The listing builds one solid part. Answer for the finished solid, in the listing's coordinates (mm). Face numbers are marked on the shaded views. A direction names the side the tool comes from. Coordinates: 2 decimals unless noted, no trailing zeros. Order: outer loops, then holes, each group sorted by start corner. A loop starts at its lowest first (then second) coordinate and runs counter-clockwise, first axis right, second up.
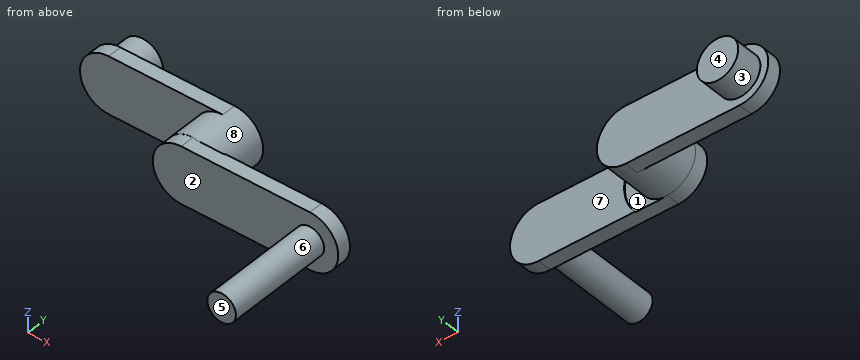
from build123d import *

# Parameters (mm, degrees)
SKETCH1_R           = 30
BOSS_EXTRUDE1_DEPTH = 25.4
BOSS_EXTRUDE2_DEPTH = 10
SKETCH3_R           = 14.5
BOSS_EXTRUDE3_DEPTH = 18.864779219
BOSS_EXTRUDE4_DEPTH = 10
SKETCH5_R           = 10
BOSS_EXTRUDE5_DEPTH = 75
CUT_EXTRUDE1_START  = -26
SKETCH7_R           = 30
SKETCH7_R_2         = 20
CUT_EXTRUDE1_DEPTH  = 26


with BuildPart() as part:
    # Sketch1 → Boss-Extrude1 (new body)
    with BuildSketch(Plane(origin=(0, 0, 0), x_dir=(1, 0, 0), z_dir=(0, 1, 0))):
        with Locations(Location((0, 0, 0), (0, 0, 270))):
            Circle(SKETCH1_R)
    extrude(amount=BOSS_EXTRUDE1_DEPTH)

    # Sketch2 → Boss-Extrude2 (add)
    with BuildSketch(Plane(origin=(0, 25.4, 0), x_dir=(1, 0, 0), z_dir=(0, 1, 0))):
        with BuildLine():
            Line((0, -20), (-80, -20))
            ThreePointArc((-80, -20), (-100, 0), (-80, 20))
            Line((-80, 20), (0, 20))
            ThreePointArc((0, 20), (20, 0), (0, -20))
        make_face()
    extrude(amount=BOSS_EXTRUDE2_DEPTH)

    # Sketch3 → Boss-Extrude3 (add)
    with BuildSketch(Plane(origin=(0, 35.4, 0), x_dir=(1, 0, 0), z_dir=(0, 1, 0))):
        with Locations(Location((-80, 0, 0), (0, 0, 270))):
            Circle(SKETCH3_R)
    extrude(amount=BOSS_EXTRUDE3_DEPTH)

    # Sketch4 → Boss-Extrude4 (add)
    with BuildSketch(Plane.XZ):
        with BuildLine():
            Line((0, 19.919861454), (90, 19.919861454))
            ThreePointArc((90, 19.919861454), (109.919861454, 0), (90, -19.919861454))
            Line((90, -19.919861454), (0, -19.919861454))
            ThreePointArc((0, -19.919861454), (-19.919861454, 0), (0, 19.919861454))
        make_face()
    extrude(amount=BOSS_EXTRUDE4_DEPTH)

    # Sketch5 → Boss-Extrude5 (add)
    with BuildSketch(Plane.XZ.offset(10)):
        with Locations(Location((90, 0, 0), (0, 0, 270))):
            Circle(SKETCH5_R)
    extrude(amount=BOSS_EXTRUDE5_DEPTH)

    # Sketch7 → Cut-Extrude1 (cut)
    with BuildSketch(Plane(origin=(0, 25.4, 0), x_dir=(1, 0, 0), z_dir=(0, 1, 0)).offset(CUT_EXTRUDE1_START)):
        Circle(SKETCH7_R)
        with Locations(Location((0, 0, 0), (0, 0, 90))):
            Circle(SKETCH7_R_2, mode=Mode.SUBTRACT)
    extrude(amount=CUT_EXTRUDE1_DEPTH, mode=Mode.SUBTRACT)


solid = part.part
(1) Find the intervals of material crossed by probe 1 along Y at (x, z) = (-2, 12); probe 2 along Y at (x, z) = (86.5, -10); probe 3 along X at (y, z) = (-76, -0.5), in increasing order.
(2) Find section C-C on y = 21. Determine the outline of the cut face in (x, z).
(3) Find section A-A on z = 0. Determine the outline of the cut face in (x, y), then the cut area to 3 significant figures.
(4) A tool of negligible diameter and unlimited length cuts with its end or side. For the marked faces 4, 5, 6, 7 and 8, from which of +Z, -Z, +X, -X, +Y, -Y can it reach the whole face along a straight path? Write none if from no direction.
(5) Given pin 1 Ø8 at (y, z) = (-35, -11.5) entering from -X; pin 2 Ø12 at (x, z) = (70, -5.5) entering from -Y; pin 3 Ø12 at (x, z) = (-74, 6.5) entering from -Y, each flat-ended and moving along its own axis, determine where each tip first touches the part or whether it passes through.
(6) The mould has two halves that part along X. Classify the marked faces 1, 2 and 3: pulls with the +X half, pulls with the -X half, needs draft (parallel to the pull), parting line crosses it, or undercut.
(7) Find section B-B on x = 56. Determine the outline of the cut face in (y, z), then the cut area to 3 significant figures.
(8) Find section D-D on x = -16.5. Determine the outline of the cut face in (y, z), then the cut area to 3 significant figures.
Resolved:
1. probe 1: y = -10 to 35.4
1. probe 2: y = -10 to 0
1. probe 3: x = 80.01 to 99.99
2. outline: circle Ø40 at (0, 0)
3. outline: (-100, 25.4) - (-20, 25.4) - (-20, 0) - (-19.92, 0) - (-19.92, -10) - (80, -10) - (80, -85) - (100, -85) - (100, -10) - (109.92, -10) - (109.92, 0) - (30, 0) - (30, -0.6) - (20, -0.6) - (20, 35.4) - (-65.5, 35.4) - (-65.5, 54.26) - (-94.5, 54.26) - (-94.5, 35.4) - (-100, 35.4) - close
3. area: 5,560 mm2
4. face 4: +Z, -Z, +X, -X, +Y
4. face 5: +Z, -Z, +X, -X, -Y
4. face 6: -Y
4. face 7: +Z, -Z, +X, +Y
4. face 8: none
5. pin 1: stops at x = 83.39
5. pin 2: stops at y = -10
5. pin 3: stops at y = 25.4
6. face 1: undercut
6. face 2: needs draft
6. face 3: parting line crosses it
7. outline: (-10, -19.92) - (0, -19.92) - (0, 19.92) - (-10, 19.92) - close
7. area: 398 mm2
8. outline: (-10, -11.16) - (0, -11.16) - (0, -11.3) - (25.4, -11.3) - (25.4, -20) - (35.4, -20) - (35.4, 20) - (25.4, 20) - (25.4, 11.3) - (0, 11.3) - (0, 11.16) - (-10, 11.16) - close
8. area: 1,200 mm2
